```python
from build123d import *

# Parameters (mm, degrees)
SKETCH1_R           = 0.5
SKETCH1_R_2         = 2.35
BOSS_EXTRUDE1_DEPTH = 1.5
SKETCH6_R           = 2.35
SKETCH6_R_2         = 1.275
BOSS_EXTRUDE2_DEPTH = 0.5
SKETCH6_3_R         = 3.45
SKETCH6_3_R_2       = 2.35
BOSS_EXTRUDE3_DEPTH = 2.5


with BuildPart() as part:
    # Sketch1 → Boss-Extrude1 (new body)
    with BuildSketch(Plane(origin=(0, 0, 0), x_dir=(1, 0, 0), z_dir=(0, 1, 0))):
        with BuildLine():
            Line((-1.733484834, -2.890728916), (-1.5, -6.6))
            ThreePointArc((-1.5, -6.6), (0, -8.1), (1.5, -6.6))
            Line((1.5, -6.6), (1.708462071, -3.437725396))
            Line((1.708462071, -3.437725396), (16.95, -1.5))
            ThreePointArc((16.95, -1.5), (18.45, 0), (16.95, 1.5))
            Line((16.95, 1.5), (1.708462071, 3.462274604))
            Line((1.708462071, 3.462274604), (1.5, 6.35))
            ThreePointArc((1.5, 6.35), (0, 7.85), (-1.5, 6.35))
            Line((-1.5, 6.35), (-1.733484834, 2.909271084))
            Line((-1.733484834, 2.909271084), (-14.35, 1.5))
            ThreePointArc((-14.35, 1.5), (-15.85, 0), (-14.35, -1.5))
            Line((-14.35, -1.5), (-1.733484834, -2.890728916))
        make_face()
        with Locations((0, -4.6)):
            Circle(SKETCH1_R, mode=Mode.SUBTRACT)
        with Locations((0, -6.6)):
            Circle(SKETCH1_R, mode=Mode.SUBTRACT)
        Circle(SKETCH1_R_2, mode=Mode.SUBTRACT)
        with Locations((16.95, 0)):
            Circle(SKETCH1_R, mode=Mode.SUBTRACT)
        with Locations((12.95, 0)):
            Circle(SKETCH1_R, mode=Mode.SUBTRACT)
        with Locations((14.95, 0)):
            Circle(SKETCH1_R, mode=Mode.SUBTRACT)
        with Locations((10.95, 0)):
            Circle(SKETCH1_R, mode=Mode.SUBTRACT)
        with Locations((8.95, 0)):
            Circle(SKETCH1_R, mode=Mode.SUBTRACT)
        with Locations((6.95, 0)):
            Circle(SKETCH1_R, mode=Mode.SUBTRACT)
        with Locations((4.95, 0)):
            Circle(SKETCH1_R, mode=Mode.SUBTRACT)
        with Locations((-14.35, 0)):
            Circle(SKETCH1_R, mode=Mode.SUBTRACT)
        with Locations((-12.35, 0)):
            Circle(SKETCH1_R, mode=Mode.SUBTRACT)
        with Locations((-10.35, 0)):
            Circle(SKETCH1_R, mode=Mode.SUBTRACT)
        with Locations((-8.35, 0)):
            Circle(SKETCH1_R, mode=Mode.SUBTRACT)
        with Locations((-6.35, 0)):
            Circle(SKETCH1_R, mode=Mode.SUBTRACT)
        with Locations((-4.35, 0)):
            Circle(SKETCH1_R, mode=Mode.SUBTRACT)
        with Locations((0, 6.35)):
            Circle(SKETCH1_R, mode=Mode.SUBTRACT)
        with Locations((0, 4.35)):
            Circle(SKETCH1_R, mode=Mode.SUBTRACT)
    extrude(amount=BOSS_EXTRUDE1_DEPTH)

    # Sketch6 → Boss-Extrude2 (add)
    with BuildSketch(Plane(origin=(0, 1.5, 0), x_dir=(1, 0, 0), z_dir=(0, 1, 0))):
        Circle(SKETCH6_R)
        Circle(SKETCH6_R_2, mode=Mode.SUBTRACT)
    extrude(amount=-BOSS_EXTRUDE2_DEPTH)

    # Sketch6_3 → Boss-Extrude3 (add)
    with BuildSketch(Plane(origin=(0, 1.5, 0), x_dir=(1, 0, 0), z_dir=(0, 1, 0))):
        Circle(SKETCH6_3_R)
        Circle(SKETCH6_3_R_2, mode=Mode.SUBTRACT)
    extrude(amount=BOSS_EXTRUDE3_DEPTH)


solid = part.part
```
Check sheet for the modelled part. Datum: model origin and axes. Units: mm. A direction names the side the tool comes from. Round coordinates to 2 decimals unless told otherwise and drop trailing zeros. Loops run counter-clockwise (first coordinate to the right, second up) from the corner with the lowest first, then second, coordinate; pieces in that order, holes last. Notation, with made-up numbers: M 3,81.5 L 57,81.5 A25 ccw 57,96.5 Z; hole C 70,-35.75 d8. An arc over 180 degrees is marked long. Answer as a JSON object with one key per item and string values.
1. Gauge pin test, flat ends, axial feed: P1, Ø3, axis at x = -12, z = 0.5, coming from the +Y side; P2, Ø6, axis at x = 9.5, z = 2, coming from the -Y side. Record the tip position at first contact, or that the pin passes through.
Reply:
{"P1": "stops at y = 1.5", "P2": "stops at y = 0"}
2. Section check C-C (x = 6.95). Record the boundary of the cut face in (y, z).
Reply:
{"outline": "M 0,-2.79 L 1.5,-2.79 L 1.5,-0.5 L 0,-0.5 Z; M 0,0.5 L 1.5,0.5 L 1.5,2.77 L 0,2.77 Z"}
3. Section check D-D (x = 3). Record the boundary of the cut face in (y, z).
Reply:
{"outline": "M 0,-3.3 L 1.5,-3.3 L 1.5,-1.7 L 4,-1.7 L 4,1.7 L 1.5,1.7 L 1.5,3.27 L 0,3.27 Z"}
4. Mould release check, pull along Z, two halves, no side actions. Record for faces 4 (the cylindrical face through (0, 0.7, 8.1)), 5 (the cylindrical face through (-0.065, 0.74, -6.846)), 6 (the flat face through (2.5, 0, 0.7)): pulls with the +Z half, pulls with the -Z half, needs draft (parallel to the pull), parting line crosses it, or undercut.
Reply:
{"face 4": "pulls with the +Z half", "face 5": "undercut", "face 6": "needs draft"}
5. Section check A-A (y = 0.4). State how many separate pieces and enclosed holes the cut face has, plus the area to 3 significant figures.
Reply:
{"separate pieces": "1", "enclosed holes": "18", "area": "158 mm²"}
6. Access from +Z, -Z, +X, -X, +Y, -Y to the whole of each face (thin tool, end or side, straight path). Record for faces 1 (the cylindrical face through (-0.509, 2.732, 2.294)), 2 (the cylindrical face through (-0.509, 0.493, 2.294)), 3 (the flat face through (9.223, 0.74, 2.482)).
Reply:
{"face 1": "+Y", "face 2": "-Y", "face 3": "+Z, +X, +Y, -Y"}
7. Scan lines: line 1 (Z direction, x = 16.95, y = 1.1); line 2 (Z direction, x = 0, y = 0.95); line 3 (Y direction, x = -1, z = 1.5). Record each from-to range of solid material in increasing order.
Reply:
{"line 1": "z = -1.5 to -0.5, 0.5 to 1.5", "line 2": "z = -7.85 to -6.85, -5.85 to -4.85, -3.85 to -2.35, 2.35 to 4.1, 5.1 to 6.1, 7.1 to 8.1", "line 3": "y = 1 to 1.5"}
8. Section check B-B (z = -4.35). Record the boundary of the cut face in (x, y), plus the area to 3 significant figures.
Reply:
{"outline": "M -1.64,0 L -0.5,0 L -0.5,1.5 L -1.64,1.5 Z; M 0.5,0 L 1.64,0 L 1.64,1.5 L 0.5,1.5 Z", "area": "3.42 mm²"}
